Work out the finished part from the listing and answer in its coordinate system (mm). A direction names the side the tool comes from. Coordinates: 2 decimals unless noted, no trailing zeros. Loops run counter-clockwise (first coordinate to the right, second up) from the corner with the lowest first, then second, coordinate; pieces in that order, holes last. Notation, with made-up numbers: (58.5, -25) - (107.5, -25) arc R25 cw to (107.5, 13) - close; hole circle Ø11 at (-9.75, -37.75). An arc over 180 degrees is marked (long way). Write each question's results on one line, items separated by ' | '. Start each with the question number.
Item 1: Section A-A, the plane x = 10.5 is taken. Write down the section's boundary in (y, z), plus the area to 3 significant figures.
Item 2: Section C-C, the plane z = 0.3 is taken. Write down the section's boundary in (x, y), plus the area to 3 significant figures.
Item 3: Each of these flat-tipped pins is pushed along its axis until it touches: pin 1 Ø6 at (x, y) = (-6, 62.5) entering from -Z; pin 2 Ø6 at (x, y) = (-1.5, 8) entering from -Z; pin 3 Ø6 at (x, y) = (14.5, 60.5) entering from -Z; pin 4 Ø10.5 at (x, y) = (10.5, 7) entering from +Z. Where does it stop, or does it pass through?
Item 4: Section B-B, the plane y = 22 is taken. Write down the section's boundary in (x, z).
Item 5: Section D-D, the plane x = -1 is taken. Write down the section's boundary in (y, z).
Item 6: A tool of negligible diameter and unlimited length cuts with its end or side. For faces 4 (the face through (0, 30, -0.75)), 5 (the face through (13.8, 7.1, 0)), from which of +Z, -Z, +X, -X, +Y, -Y can it reach the whole face along a straight path? Write none if from no direction.
Item 7: For a pull along Y with two mould halves and no side action, classify faces 1 (the face through (13.119, 19.992, -0.011)), 2 (the face through (18.574, 73.568, -1.174)), 3 (the face through (0, 30, 0.75)) as +Y half, -Y half, draft (parallel to the pull), parting line (faces both ways), or undercut.
Item 8: Consider probe 1 along Z at (x, y) = (3, 45.5); probe 2 along Y at (x, z) = (17, -0.6); probe 3 along Z at (x, y) = (-3.5, 65). Determine where each line is inside the solid, lowest interval first. Write a range as [from, to].
from build123d import *

# Parameters (mm, degrees)
F1_DEPTH = 20
F3_D     = 6.6
F3_DEPTH = 43
F3_TIP   = 1.9828400428
F4_R     = 5


with BuildPart() as f1:
    # F0 (on Right) → F1 (new body, symmetric)
    with BuildSketch(Plane.YZ):
        Polygon((0, 0), (0, -0.75), (60, -0.75), (75, -2.0623299529), (75.1307336141, -0.5680379058), (60.0654914144, 0.75), (0, 0.75), align=None)
    extrude(amount=F1_DEPTH, both=True)

    # F3
    with Locations(Plane.XY.offset(0.75)):
        with Locations((-10.5, 7), (10.5, 7), (10.5, 22), (-10.5, 22)):
            Hole(F3_D / 2, depth=F3_DEPTH)
            with Locations((0, 0, -(F3_DEPTH + F3_TIP / 2))):  # 118° drill point
                Cone(0, F3_D / 2, F3_TIP, mode=Mode.SUBTRACT)

    # F4
    f4_edges = [f1.edges().sort_by_distance(p)[0] for p in [
        (20, 75.065367, -1.315184),
        (-20, 75.065367, -1.315184),
        (20, 0, 0),
        (-20, 0, 0),
    ]]
    fillet(f4_edges, radius=F4_R)


solid = f1.part
Answer key:
1) outline: (0, -0.75) - (3.7, -0.75) - (3.7, 0.75) - (0, 0.75) - close; (10.3, -0.75) - (18.7, -0.75) - (18.7, 0.75) - (10.3, 0.75) - close; (25.3, -0.75) - (60, -0.75) - (75, -2.06) - (75.13, -0.57) - (60.07, 0.75) - (25.3, 0.75) - close | area: 92.9 mm^2
2) outline: (-20, 5) arc R5 ccw to (-15, 0) - (15, 0) arc R5 ccw to (20, 5) - (20, 65.21) - (-20, 65.21) - close; hole circle Ø6.6 at (-10.5, 7); hole circle Ø6.6 at (-10.5, 22); hole circle Ø6.6 at (10.5, 7); hole circle Ø6.6 at (10.5, 22) | area: 2,460 mm^2
3) pin 1: stops at z = -1.23 | pin 2: stops at z = -0.75 | pin 3: stops at z = -1.06 | pin 4: stops at z = 0.75
4) outline: (-20, -0.75) - (-13.8, -0.75) - (-13.8, 0.75) - (-20, 0.75) - close; (-7.2, -0.75) - (7.2, -0.75) - (7.2, 0.75) - (-7.2, 0.75) - close; (13.8, -0.75) - (20, -0.75) - (20, 0.75) - (13.8, 0.75) - close
5) outline: (0, -0.75) - (60, -0.75) - (75, -2.06) - (75.13, -0.57) - (60.07, 0.75) - (0, 0.75) - close
6) face 4: -Z, +X, -X, -Y | face 5: +Z, -Z
7) face 1: undercut | face 2: +Y half | face 3: draft
8) probe 1: z = [-0.75, 0.75] | probe 2: y = [0.42, 74.71] | probe 3: z = [-1.19, 0.32]
